Drawing for the job (mm, zero at the part's lowest x, y, z). A direction names the side the tool comes from. Coordinates: 2 decimals unless noted, no trailing zeros. Loops run counter-clockwise (first coordinate to the right, second up) from the corner with the lowest first, then second, coordinate; pieces in that order, holes last. Notation, with made-up numbers: (37.5, -11.75) - (95.5, -11.75) arc R14 cw to (95.5, -7.75) - close; hole circle Ø3 at (72.25, 45). An arc over 180 degrees is marked (long way). One line per item, written item: value.
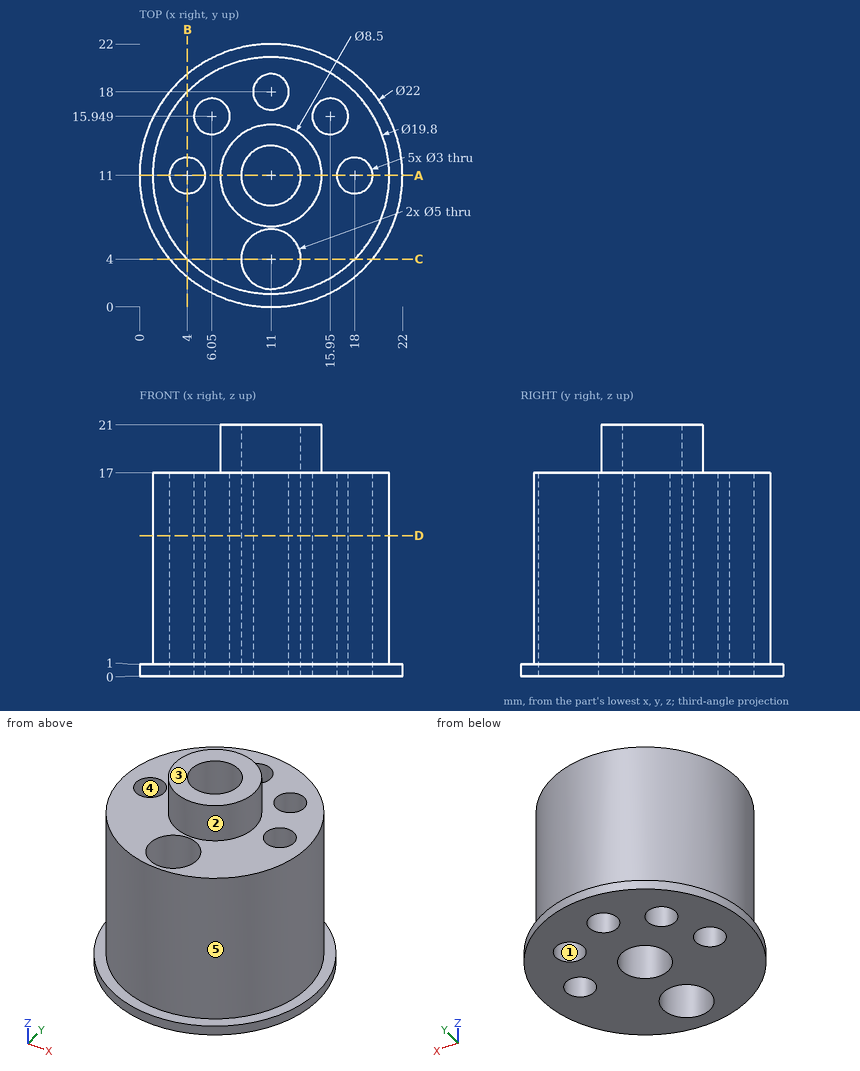
Item 1: Cut at B-B, the plane x = 4. Write the cut outline in (y, z) (1 decimal), then the cut area to 3 significant figures.
Check result:
outline: (2.5, 0) - (9.5, 0) - (9.5, 17) - (4, 17) - (4, 1) - (2.5, 1) - close; (12.5, 0) - (19.5, 0) - (19.5, 1) - (18, 1) - (18, 17) - (12.5, 17) - close
area: 190 mm^2
Item 2: Cut at D-D, the plane z = 11.75. Write the cut outline in (x, y), then the cut area to 3 significant figures.
Check result:
outline: circle Ø19.8 at (11, 11); hole circle Ø3 at (4, 11); hole circle Ø3 at (6.05, 15.95); hole circle Ø5 at (11, 4); hole circle Ø5 at (11, 11); hole circle Ø3 at (11, 18); hole circle Ø3 at (15.95, 15.95); hole circle Ø3 at (18, 11)
area: 233 mm^2
Item 3: Probe probe 1 along Y at (x, z) = (11, 8.5); probe 2 along Y at (x, z) = (16.75, 6.5) (1 decimal); probe 3 along Z at (x, y) = (17.5, 15). List the from-to ranges inside material, lowest first. Write a range as from..to.
Check result:
probe 1: y = 1.1..1.5, 6.5..8.5, 13.5..16.5, 19.5..20.9
probe 2: y = 2.9..10.2, 11.8..14.7, 17.2..19.1
probe 3: z = 0..17
Item 4: Tool access for the marked faces 1 and 2: list every direction of +Z, -Z, +X, -X, +Y, -Y with a clear straight run to the whole face (end or side of a thin tool).
Check result:
face 1: +Z, -Z
face 2: +Z
Item 5: Pull direction Y, two halves, no side cores. Call the marked faces 3, 4 and 5: released by +Y, released by -Y, zero draft, split by the parting line, or undercut.
Check result:
face 3: zero draft
face 4: undercut
face 5: split by the parting line
Item 6: Cut at C-C, the plane y = 4. Write the cut outline in (x, z) (1 decimal).
Check result:
outline: (2.5, 0) - (8.5, 0) - (8.5, 17) - (4, 17) - (4, 1) - (2.5, 1) - close; (13.5, 0) - (19.5, 0) - (19.5, 1) - (18, 1) - (18, 17) - (13.5, 17) - close
Item 7: Drop flat-ended pins along their axis: P1, Ø1, axis at y = 4.5, z = 13, coming from the -X side (1 decimal); P2, Ø5, axis at x = 2.5, z = 17.5, coming from the +Y side (1 decimal); P3, Ø2, axis at x = 4, z = 6, coming from the +Y side (1 decimal). Give the stop position or say it passes through.
Check result:
P1: stops at x = 3.1
P2: stops at y = 18.8
P3: stops at y = 18.9
Item 8: Cut at A-A, the plane y = 11. Write the cut outline in (x, z).
Check result:
outline: (0, 0) - (2.5, 0) - (2.5, 17) - (1.1, 17) - (1.1, 1) - (0, 1) - close; (5.5, 0) - (8.5, 0) - (8.5, 21) - (6.75, 21) - (6.75, 17) - (5.5, 17) - close; (13.5, 0) - (16.5, 0) - (16.5, 17) - (15.25, 17) - (15.25, 21) - (13.5, 21) - close; (19.5, 0) - (22, 0) - (22, 1) - (20.9, 1) - (20.9, 17) - (19.5, 17) - close
